Could you check a few things on this drawing? It's one solid part, dimensions in mm from its lowest x, y, z. Round coordinates to 2 decimals unless told otherwise and drop trailing zeros. Loops run counter-clockwise (first coordinate to the right, second up) from the corner with the lowest first, then second, coordinate; pieces in that order, holes last. Notation, with made-up numbers: M 48.5,-29.75 L 63.5,-29.75 A9 cw 63.5,-15.75 Z; hole C 58.25,65 d9. An arc over 180 degrees is marked long. Answer as a JSON object with one key per item and string values.
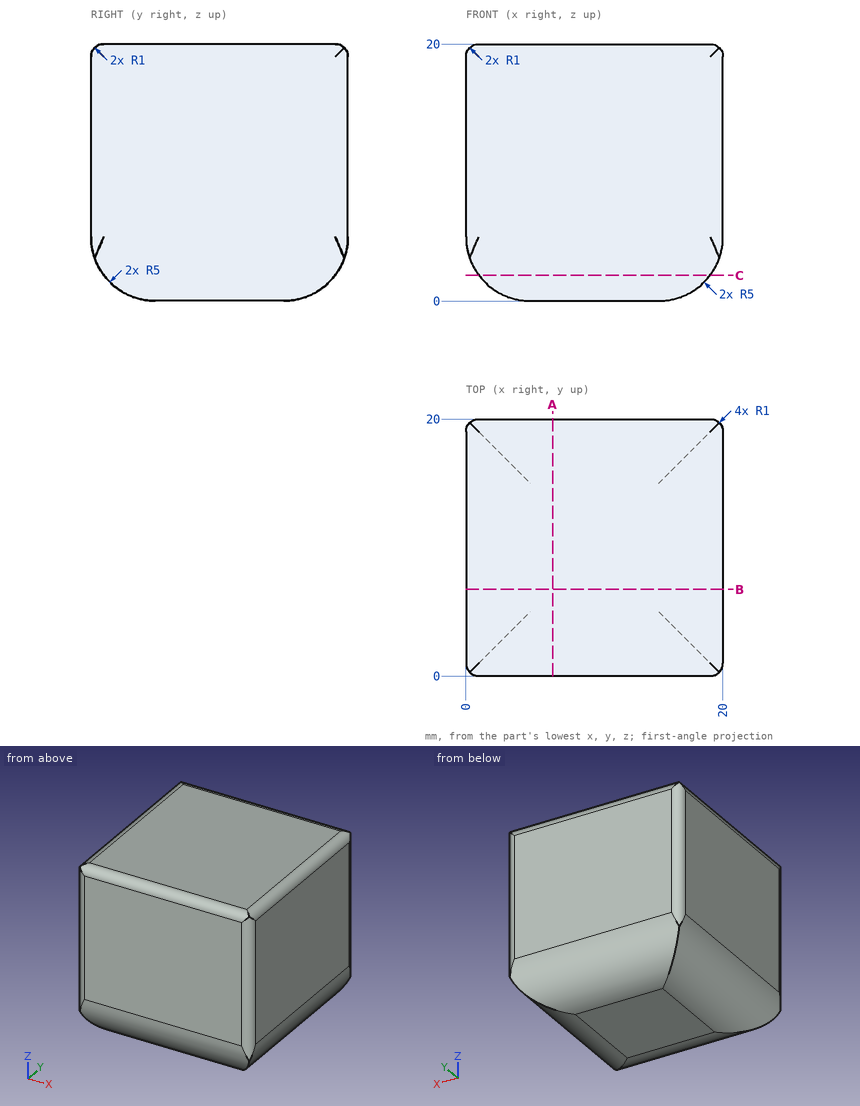
Item 1: I want a section at C-C, the plane z = 2. Please give me the cut outline in (x, y).
Resolved:
{"outline": "M 1,1 L 19,1 L 19,19 L 1,19 Z"}
Item 2: I want a section at A-A, the plane x = 6.75. Please give me the cut outline in (y, z).
Resolved:
{"outline": "M 0,5 A5 ccw 5,0 L 15,0 A5 ccw 20,5 L 20,19 A1 ccw 19,20 L 1,20 A1 ccw 0,19 Z"}
Item 3: Please list where these lines run through material, in increasing order: probe 1 along Y at (x, z) = (10, 1.5); probe 2 along X at (y, z) = (8, 4.5); probe 3 along Z at (x, y) = (17.25, 10.75). Write a range as from..to.
Resolved:
{"probe 1": "1.43..18.57", "probe 2": "0.03..19.97", "probe 3": "0.53..20"}
